from build123d import *
from build123d.topology import SkipClean

# Parameters (mm, degrees)
EXTRUDE_1_DEPTH     = 3
SKETCH_2_R          = 3
EXTRUDE_2_DEPTH     = 0.5
SKETCH_3_R          = 3
EXTRUDE_3_DEPTH     = 3
SKETCH_4_R          = 1.75
CUT_EXTRUDE_1_DEPTH = 36.833503876


with BuildPart() as part:
    # Sketch 1 → Extrude 1 (new body)
    with BuildSketch(Plane(origin=(0, 0, 0), x_dir=(1, 0, 0), z_dir=(0, 1, 0))):
        with BuildLine():
            Line((0, 3), (32.2, 3))
            ThreePointArc((32.2, 3), (35.2, 0), (32.2, -3))
            Line((32.2, -3), (0, -3))
            ThreePointArc((0, -3), (-3, 0), (0, 3))
        make_face()
    extrude(amount=EXTRUDE_1_DEPTH)

    # Sketch 2 → Extrude 2 (add)
    with SkipClean():  # the faces are left unmerged after this step: merging them gives an invalid solid
        with BuildSketch(Plane(origin=(0, 3, 0), x_dir=(1, 0, 0), z_dir=(0, 1, 0))):
            with Locations(Location((32.2, 0, 0), (0, 0, 270))):
                Circle(SKETCH_2_R)
        extrude(amount=EXTRUDE_2_DEPTH)
    add(part.part.scale(1), mode=Mode.REPLACE)  # the faces are merged on a copy

    # Sketch 3 → Extrude 3 (add)
    with SkipClean():  # the faces are left unmerged after this step: merging them gives an invalid solid
        with BuildSketch(Plane(origin=(0, 3, 0), x_dir=(1, 0, 0), z_dir=(0, 1, 0))):
            with Locations(Location((0, 0, 0), (0, 0, 270))):
                Circle(SKETCH_3_R)
        extrude(amount=EXTRUDE_3_DEPTH)

    # Sketch 4 → Cut-Extrude 1 (cut, through all)
    with SkipClean():  # the faces are left unmerged after this step: merging them gives an invalid solid
        with BuildSketch(Plane(origin=(0, 6, 0), x_dir=(1, 0, 0), z_dir=(0, 1, 0))):
            with Locations(Location((0, 0, 0), (0, 0, 270))):
                Circle(SKETCH_4_R)
            with Locations(Location((32.2, 0, 0), (0, 0, 270))):
                Circle(SKETCH_4_R)
        extrude(amount=-CUT_EXTRUDE_1_DEPTH, mode=Mode.SUBTRACT)


solid = part.part
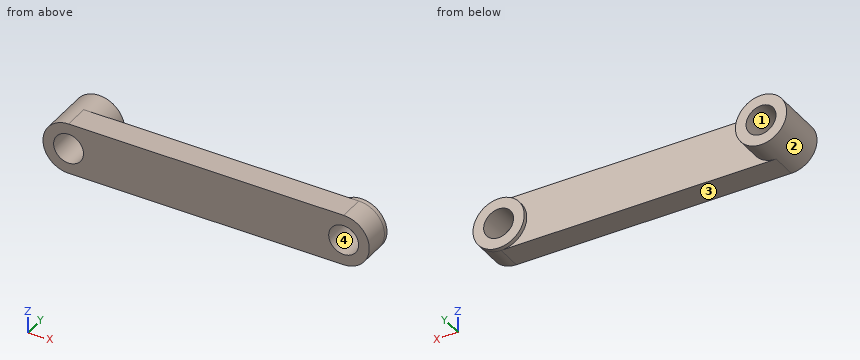
Could you check a few things on this model? Use its own coordinates, in mm. Face numbers are marked on the shaded views. A direction names the side the tool comes from. Coordinates: 2 decimals unless noted, no trailing zeros. Order: outer loops, then holes, each group sorted by start corner. A loop starts at its lowest first (then second) coordinate and runs counter-clockwise, first axis right, second up. Notation, with made-up numbers: (-31.75, 75) - (6.25, 75) arc R21 ccw to (6.25, 104) - close; hole circle Ø4 at (30.5, 74). An arc over 180 degrees is marked (long way). Answer in a Markdown table with one row per item. Add a question column.
(1) On a 3-axis mill with a long thin cutter (end or side, diameter ignored), from which of +Z, -Z, +X, -X, +Y, -Y can I reach the whole of each face in a straight line? I mean the marked faces 1 and 2. Say none if no direction works.
(2) I need wall thicknesses on L1, parallel to X at y = 2.4, z = 0; L2, parallel to X at y = 1.65, z = 0.8; L3, parallel to Y at x = 11, z = 0.4. Which ranges of each line are inside material? Lowest first, please.
(3) If we section it at D-D, the plane x = 1: Please give me the cut outline in (y, z).
(4) If we section it at A-A, the plane z = 0: Please give me the cut outline in (x, y), then the cut area to 3 significant figures.
(5) If we section it at C-C, the plane y = 5.4: Please give me the cut outline in (x, z).
(6) If we section it at B-B, the plane y = 2.55: Please give me the cut outline in (x, z), then the cut area to 3 significant figures.
(7) Will these pins go through, and if not, where does the flat tip stop? pin 1 (1.5 mm diameter, centred on y = 1, z = 2, fed in from -X); pin 2 (1.8 mm diameter, centred on x = 33.5, z = 1, fed in from +Y); pin 3 (1.5 mm diameter, centred on x = 27.5, z = -0.5, fed in from +Y).
(8) If we mould it in two halves opening along X, with no side actions, what happens to the marked faces 3 and 4? For each: released by +X, released by -X, zero draft, split by the parting line, or undercut.
Results are:
| question | item | result |
|---|---|---|
| 1 | face 1 | +Y, -Y |
| 1 | face 2 | +Y |
| 2 | L1 | x = -3 to -1.75, 1.75 to 30.45, 33.95 to 35.2 |
| 2 | L2 | x = -2.89 to -1.56, 1.56 to 30.64, 33.76 to 35.09 |
| 2 | L3 | y = 0 to 3 |
| 3 | outline | (0, -3) - (3, -3) - (3, -2.83) - (6, -2.83) - (6, -1.44) - (0, -1.44) - close; (0, 1.44) - (6, 1.44) - (6, 2.83) - (3, 2.83) - (3, 3) - (0, 3) - close |
| 4 | outline | (-3, 0) - (-1.75, 0) - (-1.75, 6) - (-3, 6) - close; (1.75, 0) - (30.45, 0) - (30.45, 3.5) - (29.2, 3.5) - (29.2, 3) - (3, 3) - (3, 6) - (1.75, 6) - close; (33.95, 0) - (35.2, 0) - (35.2, 3.5) - (33.95, 3.5) - close |
| 4 | area | 102 mm2 |
| 5 | outline | circle Ø6 at (0, 0); hole circle Ø3.5 at (0, 0) |
| 6 | outline | (0, -3) - (32.2, -3) arc R3 ccw to (32.2, 3) - (0, 3) arc R3 ccw to start; hole circle Ø3.5 at (0, 0); hole circle Ø3.5 at (32.2, 0) |
| 6 | area | 202 mm2 |
| 7 | pin 1 | stops at x = -2.73 |
| 7 | pin 2 | stops at y = 3.5 |
| 7 | pin 3 | stops at y = 3 |
| 8 | face 3 | zero draft |
| 8 | face 4 | undercut |
